Drawing for the job (mm, zero at the part's lowest x, y, z). A direction names the side the tool comes from. Coordinates: 2 decimals unless noted, no trailing zeros. Order: outer loops, then holes, each group sorted by start corner. A loop starts at its lowest first (then second) coordinate and runs counter-clockwise, first axis right, second up.
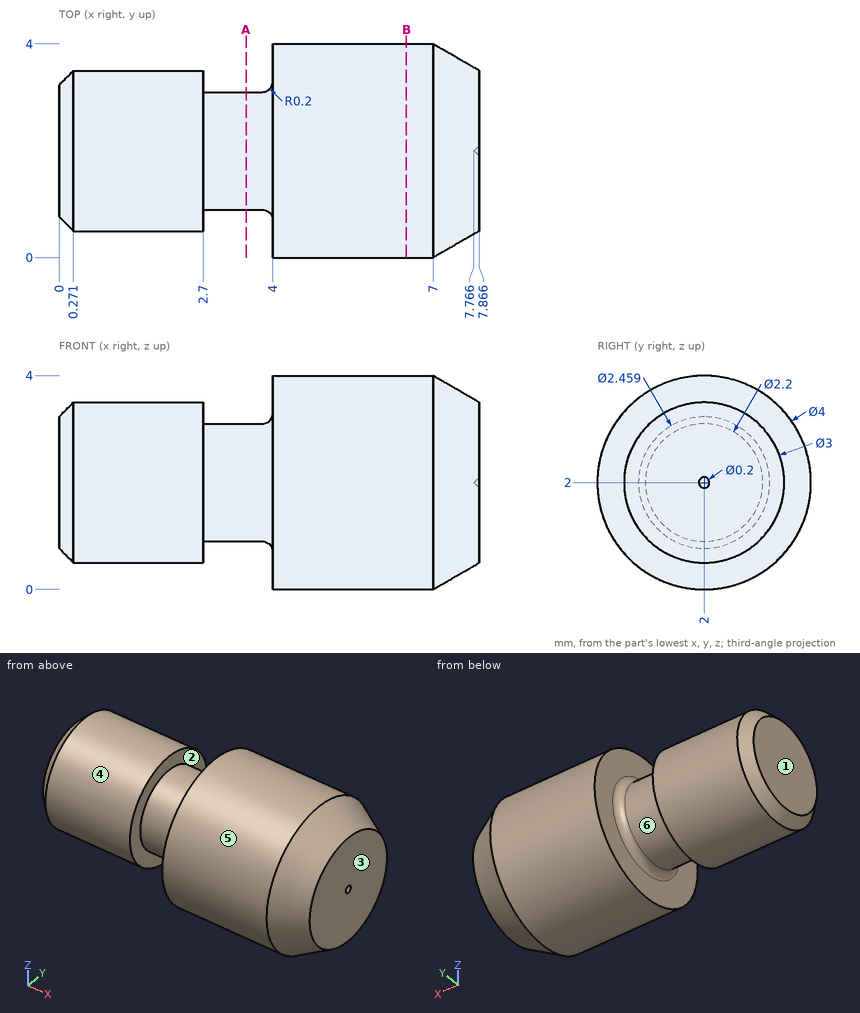
1) Drill centre lines: probe 1 along X at (y, z) = (2.3, 3.4) (1 decimal); probe 2 along Y at (x, z) = (5.75, 1.8); probe 3 along X at (y, z) = (2.4, 3.65) (1 decimal). Where is each one in solid material? Low to high.
2) Slice it at B-B (x = 6.5). List the corners of the cut face in (y, z).
3) Pin check, flat tips, straight feed: P1, Ø1.5, axis at x = 2.5, z = 3, coming from the +Y side; P2, Ø1, axis at x = 2.5, y = 0.5, coming from the +Z side. Stop position of each tip, or through.
4) Two-plate mould, pull along X, no slides. Class the marked faces 1, 2, 3 and 4: released by +X, released by -X, zero draft, split by the parting line, or undercut.
5) Which spindle directions (+Z, -Z, +X, -X, +Y, -Y) get a long thin tool onto all of the face, cutting with end or side? Do the marked faces 5 and 6. Say none if no direction does.
6) Slice it at A-A (x = 3.5). List the corners of the cut face in (y, z).
Worked out:
1. probe 1: x = 0.2 to 2.7, 4 to 7.9
1. probe 2: y = 0.01 to 3.99
1. probe 3: x = 4 to 7.5
2. outline: circle Ø4 at (2, 2)
3. P1: stops at y = 3.48
3. P2: stops at z = 3.12
4. face 1: released by -X
4. face 2: undercut
4. face 3: released by +X
4. face 4: zero draft
5. face 5: +X, -X
5. face 6: none
6. outline: circle Ø2.2 at (2, 2)
